from build123d import *

# Parameters (mm, degrees)
ESQUISSE1_W        = 40
ESQUISSE1_H        = 60
ESQUISSE1_R        = 1
BOSS_EXTRU_1_DEPTH = 6.5
ESQUISSE3_W        = 8
ESQUISSE3_H        = 8
ESQUISSE3_H_2      = 3
ESQUISSE3_W_2      = 2
ESQUISSE3_H_3      = 47
BOSS_EXTRU_2_DEPTH = 10


with BuildPart() as part:
    # Esquisse1 → Boss.-Extru.1 (new, symmetric)
    with BuildSketch(Plane(origin=(0, 0, 0), x_dir=(1, 0, 0), z_dir=(0, 1, 0))):
        Rectangle(ESQUISSE1_W, ESQUISSE1_H)
        with Locations(Location((-18, 28, 0), (0, 0, 90))):
            Circle(ESQUISSE1_R, mode=Mode.SUBTRACT)
        with Locations(Location((18, 28, 0), (0, 0, 90))):
            Circle(ESQUISSE1_R, mode=Mode.SUBTRACT)
        with Locations(Location((18, -28, 0), (0, 0, 90))):
            Circle(ESQUISSE1_R, mode=Mode.SUBTRACT)
        with Locations(Location((-18, -28, 0), (0, 0, 90))):
            Circle(ESQUISSE1_R, mode=Mode.SUBTRACT)
    extrude(amount=BOSS_EXTRU_1_DEPTH, both=True)

    # Esquisse3 → Boss.-Extru.2 (add)
    with BuildSketch(Plane.XZ.offset(6.5)):
        with Locations((14, 4)):
            Rectangle(ESQUISSE3_W, ESQUISSE3_H)
        with Locations((14, -5.5)):
            Rectangle(ESQUISSE3_W, ESQUISSE3_H_2)
        with Locations((9, 2.5)):
            Rectangle(ESQUISSE3_W_2, ESQUISSE3_H_3)
        with Locations((-16, 2.5)):
            Rectangle(ESQUISSE3_W_2, ESQUISSE3_H_3)
    extrude(amount=BOSS_EXTRU_2_DEPTH)


solid = part.part
Geometry check sheet. Reference: the model listing, model coordinates, mm. A direction names the side the tool comes from. Round coordinates to 2 decimals unless told otherwise and drop trailing zeros. Loops run counter-clockwise (first coordinate to the right, second up) from the corner with the lowest first, then second, coordinate; pieces in that order, holes last. Notation, with made-up numbers: (-9.5, -31) - (32.5, -31) arc R23 ccw to (32.5, -19) - close; hole circle Ø11 at (-12.75, 22). An arc over 180 degrees is marked (long way). One line per question, with ' | ' between items. Start each with the question number.
1. Tool access check on faces 4 (the face through (9, -11, 26)), 5 (the face through (14, -11, -7)), 6 (the face through (10, -11, -2)), 7 (the face through (9, -11, -21)), 8 (the face through (18, -11, -6)). Record the directions out of +Z, -Z, +X, -X, +Y, -Y that give a thin tool (end or side, any length) a straight path to the whole face; none if there is none.
2. Cross-section at B-B on z = -28. Record the cut outline in (x, y), then the cut area to 3 significant figures.
3. Depth check by flat-ended pin: pin 1 (11 mm diameter, centred on y = -14, z = -5.5, fed in from -X); pin 2 (0.6 mm diameter, centred on x = 9, y = -11.5, fed in from -Z); pin 3 (3 mm diameter, centred on y = -9.5, z = -2, fed in from +X). Enter the tip coordinate at first touch or a pass-through.
4. Draft check along X on faces 1 (the face through (-20, 0, 0)), 2 (the face through (14, -11, -4)), 3 (the face through (19, 0, 28)). Enter one of: released by +X, released by -X, zero draft, split by the parting line, or undercut.
5. Cross-section at C-C on x = 11.5. Record the cut outline in (y, z).
6. Cross-section at A-A on y = -11.5. Record the cut outline in (x, z), then the cut area to 3 significant figures.
7. Scan lines: line 1 (Z direction, x = 18, y = -4); line 2 (X direction, y = 2, z = -28); line 3 (Z direction, x = 17.5, y = 5.5). Record each from-to range of solid material in increasing order. Write a range as [from, to].
8. Cross-section at D-D on x = -18. Record the cut outline in (y, z), then the cut area to 3 significant figures.
Taken from the geometry:
1) face 4: +Z, +X, -X, -Y | face 5: -Z, +X, -Y | face 6: +X, -Y | face 7: -Z, +X, -X, -Y | face 8: +Z, -Z, +X, -Y
2) outline: (-20, -6.5) - (-19, -6.5) - (-19, 6.5) - (-20, 6.5) - close; (-17, -6.5) - (17, -6.5) - (17, 6.5) - (-17, 6.5) - close; (19, -6.5) - (20, -6.5) - (20, 6.5) - (19, 6.5) - close | area: 468 mm²
3) pin 1: x = -17 | pin 2: z = -21 | pin 3: x = 10
4) face 1: released by -X | face 2: zero draft | face 3: undercut
5) outline: (-16.5, -7) - (-6.5, -7) - (-6.5, -30) - (6.5, -30) - (6.5, 30) - (-6.5, 30) - (-6.5, 8) - (-16.5, 8) - (-16.5, 0) - (-6.5, 0) - (-6.5, -4) - (-16.5, -4) - close
6) outline: (-17, -21) - (-15, -21) - (-15, 26) - (-17, 26) - close; (8, -21) - (10, -21) - (10, -7) - (18, -7) - (18, -4) - (10, -4) - (10, 0) - (18, 0) - (18, 8) - (10, 8) - (10, 26) - (8, 26) - close | area: 276 mm²
7) line 1: [-30, -29], [-27, 27], [29, 30] | line 2: [-20, -19], [-17, 17], [19, 20] | line 3: [-30, -28.87], [-27.13, 27.13], [28.87, 30]
8) outline: (-6.5, -30) - (6.5, -30) - (6.5, -29) - (-6.5, -29) - close; (-6.5, -27) - (6.5, -27) - (6.5, 27) - (-6.5, 27) - close; (-6.5, 29) - (6.5, 29) - (6.5, 30) - (-6.5, 30) - close | area: 728 mm²
